```python
from build123d import *

# Parameters (mm, degrees)
SKETCH_R        = 1.8
PAD_DEPTH       = 6
SKETCH001_W     = 70.6
SKETCH001_H     = 55.3
POCKET_DEPTH    = 4
SKETCH002_R     = 3
PAD001_DEPTH    = 2.4
SKETCH003_R     = 1.5
PAD002_DEPTH    = 1.6
POCKET001_DEPTH = 3
POCKET002_DEPTH = 3
SKETCH006_W     = 55
SKETCH006_H     = 39
POCKET003_DEPTH = 5


with BuildPart() as part:
    # Sketch → Pad (new body)
    with BuildSketch(Plane.XY):
        with BuildLine():
            ThreePointArc((-3, 0), (-2.12132, -2.12132), (0, -3))
            Line((0, -3), (9.3, -3))
            Line((9.3, -3), (9.3, -7))
            ThreePointArc((9.3, -7), (14.3, -12), (19.3, -7))
            Line((19.3, -7), (19.3, -3))
            Line((19.3, -3), (49.3, -3))
            Line((49.3, -3), (49.3, -7))
            ThreePointArc((49.3, -7), (54.3, -12), (59.3, -7))
            Line((59.3, -7), (59.3, -3))
            Line((59.3, -3), (68.6, -3))
            ThreePointArc((68.6, -3), (70.72132, -2.12132), (71.6, 0))
            Line((71.6, 0), (71.6, 53.3))
            ThreePointArc((71.6, 53.3), (70.72132, 55.42132), (68.6, 56.3))
            Line((59.3, 56.3), (68.6, 56.3))
            Line((59.3, 60.3), (59.3, 56.3))
            ThreePointArc((59.3, 60.3), (54.3, 65.3), (49.3, 60.3))
            Line((49.3, 56.3), (49.3, 60.3))
            Line((19.3, 56.3), (49.3, 56.3))
            Line((19.3, 60.3), (19.3, 56.3))
            ThreePointArc((19.3, 60.3), (14.3, 65.3), (9.3, 60.3))
            Line((9.3, 56.3), (9.3, 60.3))
            Line((0, 56.3), (9.3, 56.3))
            ThreePointArc((0, 56.3), (-2.12132, 55.42132), (-3, 53.3))
            Line((-3, 53.3), (-3, 0))
        make_face()
        with Locations((14.3, -7)):
            Circle(SKETCH_R, mode=Mode.SUBTRACT)
        with Locations((54.3, -7)):
            Circle(SKETCH_R, mode=Mode.SUBTRACT)
        with Locations((54.3, 60.3)):
            Circle(SKETCH_R, mode=Mode.SUBTRACT)
        with Locations((14.3, 60.3)):
            Circle(SKETCH_R, mode=Mode.SUBTRACT)
    extrude(amount=PAD_DEPTH)

    # Sketch001 → Pocket (cut)
    with BuildSketch(Plane.XY.offset(6)):
        with Locations((34.3, 26.65)):
            Rectangle(SKETCH001_W, SKETCH001_H)
    extrude(amount=-POCKET_DEPTH, mode=Mode.SUBTRACT)

    # Sketch002 → Pad001 (new body)
    with BuildSketch(Plane.XY.offset(2)):
        with Locations((15.1, 50.7)):
            Circle(SKETCH002_R)
        with Locations((14, 2.5)):
            Circle(SKETCH002_R)
        with Locations((65.9, 35.5)):
            Circle(SKETCH002_R)
        with Locations((65.9, 7.6)):
            Circle(SKETCH002_R)
    extrude(amount=PAD001_DEPTH)

    # Sketch003 → Pad002 (new body)
    with BuildSketch(Plane.XY.offset(4.4)):
        with Locations((15.1, 50.7)):
            Circle(SKETCH003_R)
        with Locations((14, 2.5)):
            Circle(SKETCH003_R)
        with Locations((65.9, 35.5)):
            Circle(SKETCH003_R)
        with Locations((65.9, 7.6)):
            Circle(SKETCH003_R)
    extrude(amount=PAD002_DEPTH)

    # Sketch004 → Pocket001 (cut)
    with BuildSketch(Plane(origin=(0, 0, 0), x_dir=(1, 0, 0), z_dir=(0, 0, -1))):
        Polygon((11.35, 5.296817), (11.35, 8.703183), (14.3, 10.406367), (17.25, 8.703183), (17.25, 5.296817), (14.3, 3.593633), align=None)
        Polygon((51.35, 5.296817), (51.35, 8.703183), (54.3, 10.406367), (57.25, 8.703183), (57.25, 5.296817), (54.3, 3.593633), align=None)
    extrude(amount=-POCKET001_DEPTH, mode=Mode.SUBTRACT)

    # Sketch005 → Pocket002 (cut)
    with BuildSketch(Plane(origin=(0, 0, 0), x_dir=(1, 0, 0), z_dir=(0, 0, -1))):
        Polygon((11.35, -62.003183), (11.35, -58.596817), (14.3, -56.893633), (17.25, -58.596817), (17.25, -62.003183), (14.3, -63.706367), align=None)
        Polygon((51.35, -62.003183), (51.35, -58.596817), (54.3, -56.893633), (57.25, -58.596817), (57.25, -62.003183), (54.3, -63.706367), align=None)
    extrude(amount=-POCKET002_DEPTH, mode=Mode.SUBTRACT)

    # Sketch006 → Pocket003 (cut)
    with BuildSketch(Plane.XY.offset(2)):
        with Locations((32.5, 26.5)):
            Rectangle(SKETCH006_W, SKETCH006_H)
    extrude(amount=-POCKET003_DEPTH, mode=Mode.SUBTRACT)


solid = part.part
```
Source: CAD feature listing. Evaluate the final solid. Frame: model axes, mm. A direction names the side the tool comes from. Round coordinates to 2 decimals unless told otherwise and drop trailing zeros. Loops run counter-clockwise (first coordinate to the right, second up) from the corner with the lowest first, then second, coordinate; pieces in that order, holes last.
(1) Section query D-D (y = 50.7). Output: boundary loops of the cut face in (x, z).
From the geometry:
outline: (-3, 0) - (71.6, 0) - (71.6, 6) - (69.6, 6) - (69.6, 2) - (18.1, 2) - (18.1, 4.4) - (16.6, 4.4) - (16.6, 6) - (13.6, 6) - (13.6, 4.4) - (12.1, 4.4) - (12.1, 2) - (-1, 2) - (-1, 6) - (-3, 6) - close
(2) Pull-direction query (Y, two-part tool) for faces 1 (the flat face through (16, -6, 3)), 2 (the flat face through (59.3, -5, 3)), 3 (the flat face through (5, -3, 3)); classes: +Y half, -Y half, draft (parallel to the pull), parting line (faces both ways), or undercut.
From the geometry:
face 1: undercut
face 2: draft
face 3: -Y half
(3) Section query A-A (y = 35.5). Output: boundary loops of the cut face in (x, z).
From the geometry:
outline: (-3, 0) - (5, 0) - (5, 2) - (-1, 2) - (-1, 6) - (-3, 6) - close; (60, 0) - (71.6, 0) - (71.6, 6) - (69.6, 6) - (69.6, 2) - (68.9, 2) - (68.9, 4.4) - (67.4, 4.4) - (67.4, 6) - (64.4, 6) - (64.4, 4.4) - (62.9, 4.4) - (62.9, 2) - (60, 2) - close
(4) Section query C-C (x = 65.9). Output: boundary loops of the cut face in (y, z), and give its area (3 significant figures).
From the geometry:
outline: (-3, 0) - (56.3, 0) - (56.3, 6) - (54.3, 6) - (54.3, 2) - (38.5, 2) - (38.5, 4.4) - (37, 4.4) - (37, 6) - (34, 6) - (34, 4.4) - (32.5, 4.4) - (32.5, 2) - (10.6, 2) - (10.6, 4.4) - (9.1, 4.4) - (9.1, 6) - (6.1, 6) - (6.1, 4.4) - (4.6, 4.4) - (4.6, 2) - (-1, 2) - (-1, 6) - (-3, 6) - close
area: 173 mm2
(5) Material intervals for probe 1 along Y at (x, z) = (54.3, 4.35); probe 2 along X at (y, z) = (-7, 4.5); probe 3 along Y at (x, z) = (22, 4.4), sorted ascending.
From the geometry:
probe 1: y = -12 to -8.8, -5.2 to -1, 54.3 to 58.5, 62.1 to 65.3
probe 2: x = 9.3 to 12.5, 16.1 to 19.3, 49.3 to 52.5, 56.1 to 59.3
probe 3: y = -3 to -1, 54.3 to 56.3
(6) Section query B-B (x = 27). Output: boundary loops of the cut face in (y, z).
From the geometry:
outline: (-3, 0) - (7, 0) - (7, 2) - (-1, 2) - (-1, 6) - (-3, 6) - close; (46, 0) - (56.3, 0) - (56.3, 6) - (54.3, 6) - (54.3, 2) - (46, 2) - close
(7) Contact query for flat-ended pins moving along their axis: pin 1 Ø1.8 at (x, z) = (64, 4) entering from +Y; pin 2 Ø1 at (x, z) = (20.5, 0.5) entering from -Y; pin 3 Ø1.5 at (y, z) = (-6.5, 1.5) entering from +X. Output: stop coordinate, or through.
From the geometry:
pin 1: stops at y = 56.3
pin 2: stops at y = -3
pin 3: stops at x = 59.3
(8) Access query for faces 4 (the flat face through (5, 26, 1)), 5 (the flat face through (12.85, 62.87, 1.48)), 6 (the cylindrical face through (62.9, 7.7, 3.2)), 7 (the flat face through (19.3, -5, 3)), 8 (the flat face through (9.3, 58, 3)). Directions: +Z, -Z, +X, -X, +Y, -Y. A direction counts if a zero-diameter tool reaches every point of the face in a straight line with its end or side. Return the directions, or none.
From the geometry:
face 4: +Z, -Z
face 5: -Z
face 6: +Z
face 7: +Z, -Z, -Y
face 8: +Z, -Z, -X, +Y
